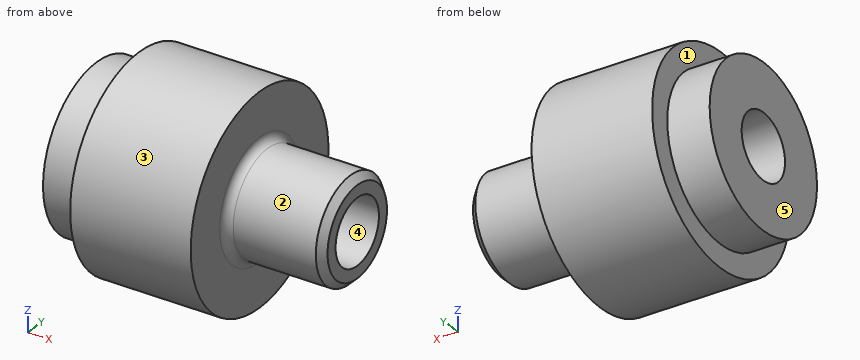
from build123d import *


# Read off the part's stored shape, not the designer's step: 1-1/4-7 Machine Threads Stud1
with BuildPart() as part:
    # Sketch1 → Revolve1 (revolve)
    with BuildSketch(Plane.XY, mode=Mode.PRIVATE) as revolve1_sk:
        with BuildLine():
            Line((-40.804054054, 10), (-27.804054054, 10))
            Line((-27.804054054, 10), (9.195945946, 10))
            Line((9.195945946, 10), (39.195945946, 10))
            Line((39.195945946, 10), (39.195945946, 15.875))
            Line((39.195945946, 15.875), (11.695945946, 15.875))
            ThreePointArc((11.695945946, 15.875), (9.928178993, 16.607233047), (9.195945946, 18.375))
            Line((9.195945946, 18.375), (9.195945946, 31.75))
            Line((9.195945946, 31.75), (-27.804054054, 31.75))
            Line((-27.804054054, 31.75), (-27.804054054, 24.75))
            Line((-27.804054054, 24.75), (-40.804054054, 24.75))
            Line((-40.804054054, 24.75), (-40.804054054, 10))
        make_face()
    revolve(revolve1_sk.sketch.rotate(Axis((-48.587837838, 0, 0), (1, 0, 0)), 90), axis=Axis((-48.587837838, 0, 0), (1, 0, 0)))

    # 1-1/4-7 Machine Threads Stud1 outline → 1-1/4-7 Machine Threads Stud1 (revolve, cut)
    with BuildSketch(Plane.YX):
        Polygon((15.875, 39.195945946), (13.71473, 39.195945946), (15.875, 37.035675946), align=None)
    revolve(axis=Axis((0, 0, 0), (1, 0, 0)), mode=Mode.SUBTRACT)


solid = part.part
Part model, mm, in its own coordinate system. Face numbers are marked on the shaded views. A direction names the side the tool comes from. Give positions to 0.01 mm unless a question says otherwise; leave off trailing zeros. Loops run counter-clockwise (first coordinate to the right, second up) from the corner with the lowest first, then second, coordinate; pieces in that order, holes last.
(1) Band-saw the part on D-D (z = -21.5). Write the cut outline in (x, y).
Return value:
outline: (-40.8, -12.26) - (-27.8, -12.26) - (-27.8, -23.36) - (9.2, -23.36) - (9.2, 23.36) - (-27.8, 23.36) - (-27.8, 12.26) - (-40.8, 12.26) - close
(2) 3-axis set-ups, long thin cutter, end or side, ignore diameter. For the marked faces 1 and 2: which of +Z, -Z, +X, -X, +Y, -Y reach the whole face in a straight line?
Return value:
face 1: -X
face 2: +X
(3) Pin check, flat tips, straight feed: pin 1 (1.5 mm diameter, centred on x = -15, z = 23, fed in from -Y); pin 2 (10 mm diameter, centred on x = 7, y = -20, fed in from +Z); pin 3 (1.5 mm diameter, centred on y = 24.5, z = 2, fed in from +X). Stop position of each tip, or through.
Return value:
pin 1: stops at y = -22.65
pin 2: stops at z = 27.98
pin 3: stops at x = 9.2
(4) Drill centre lines: line 1 along Y through (x, z) = (17, 0) (3 decimals); line 2 along Y through (x, z) = (-4.5, 0); line 3 along X through (y, z) = (-20, 16). Where is each one in solid material? Low to high.
Return value:
line 1: y = -15.875 to -10, 10 to 15.875
line 2: y = -31.75 to -10, 10 to 31.75
line 3: x = -27.8 to 9.2
(5) Band-saw the part on C-C (x = 0). Write the cut outline in (y, z).
Return value:
outline: circle Ø63.5 at (0, 0); hole circle Ø20 at (0, 0)
(6) Band-saw the part on A-A (y = 0). Write the cut outline in (x, z) (3 decimals).
Return value:
outline: (-40.804, -24.75) - (-27.804, -24.75) - (-27.804, -31.75) - (9.196, -31.75) - (9.196, -18.375) arc R2.5 cw to (11.696, -15.875) - (37.036, -15.875) - (39.196, -13.715) - (39.196, -10) - (-40.804, -10) - close; (-40.804, 10) - (39.196, 10) - (39.196, 13.715) - (37.036, 15.875) - (11.696, 15.875) arc R2.5 cw to (9.196, 18.375) - (9.196, 31.75) - (-27.804, 31.75) - (-27.804, 24.75) - (-40.804, 24.75) - close
(7) Pull direction Z, two halves, no side cores. Call the marked faces 3, 4 and 5: pulls with the +Z half, pulls with the -Z half, needs draft (parallel to the pull), parting line crosses it, or undercut.
Return value:
face 3: parting line crosses it
face 4: undercut
face 5: needs draft
